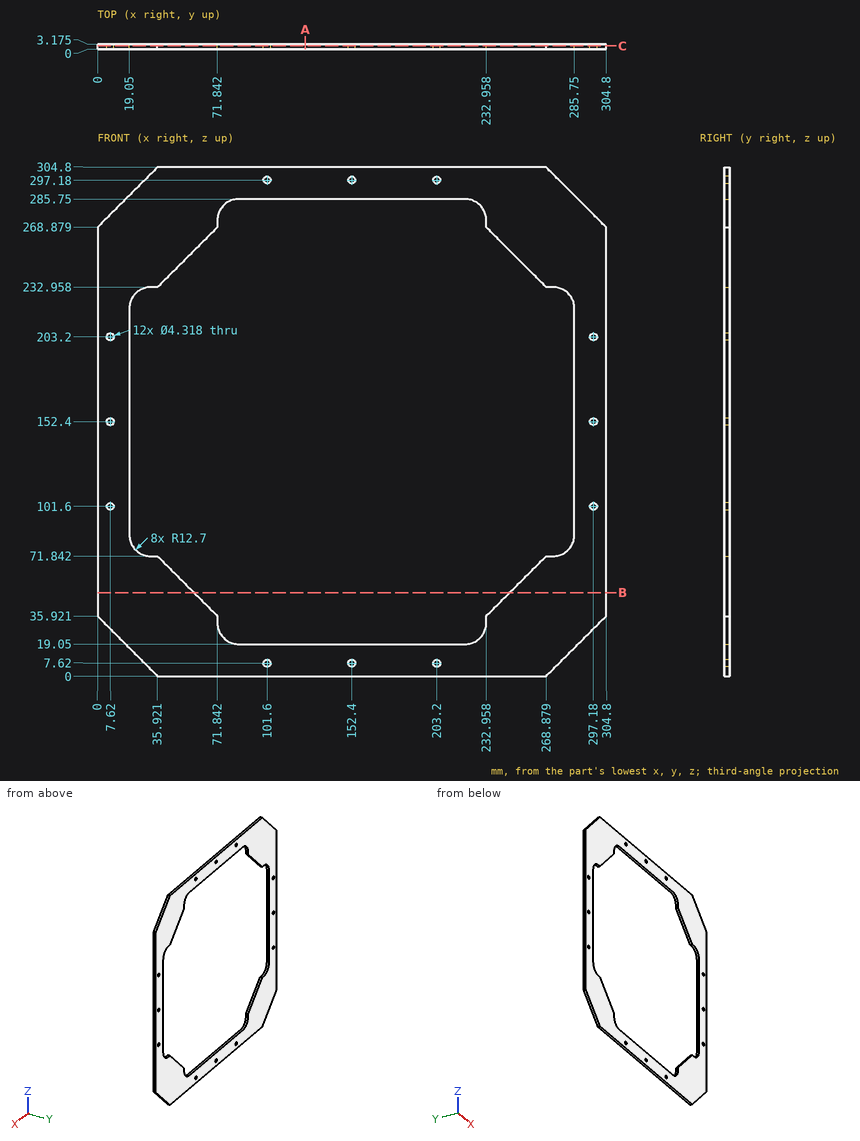
Geometry: see drawing. Coordinates: mm, zero at the bounding-box minimum. Round coordinates to 2 decimals unless told otherwise and drop trailing zeros. Write each loop counter-clockwise with the first axis right and the second up, starting at its lowest first coordinate (ties: lowest second). Pieces come first, ordered by that corner, then holes. Notation, with made-up numbers: (-27, 59) - (-17, 59) arc R10 ccw to (-17, 68) - close; hole circle Ø1 at (67, 66.5). An arc over 180 degrees is marked (long way). Use CSV: the item, a comma, the result in double quotes. Start each with the question number.
(1) Cut plane B-B, the plane z = 50. Return loops of the section in (x, y) (3 decimals), and give its area (3 significant figures).
(2) Material intervals for probe 1 along X at (y, z) = (0.75, 203.2); probe 2 along Z at (x, y) = (175, 1.1), sorted ascending. Write a range as [from, to].
(3) Cut plane A-A, the plane x = 124.5. Return loops of the section in (y, z) (3 decimals).
(4) Cut plane C-C, the plane y = 2.05. Give the number of separate pieces and of enclosed holes in the cut face, and give its area (3 significant figures).
Geometry says:
1,outline,"(0, 0) - (57.763, 0) - (57.763, 3.175) - (0, 3.175) - close; (247.037, 0) - (304.8, 0) - (304.8, 3.175) - (247.037, 3.175) - close"
1,area,"367 mm²"
2,probe 1,"[0, 5.46], [9.78, 19.05], [285.75, 295.02], [299.34, 304.8]"
2,probe 2,"[0, 19.05], [285.75, 304.8]"
3,outline,"(0, 0) - (3.175, 0) - (3.175, 19.05) - (0, 19.05) - close; (0, 285.75) - (3.175, 285.75) - (3.175, 304.8) - (0, 304.8) - close"
4,separate pieces,"1"
4,enclosed holes,"13"
4,area,"27,900 mm²"
